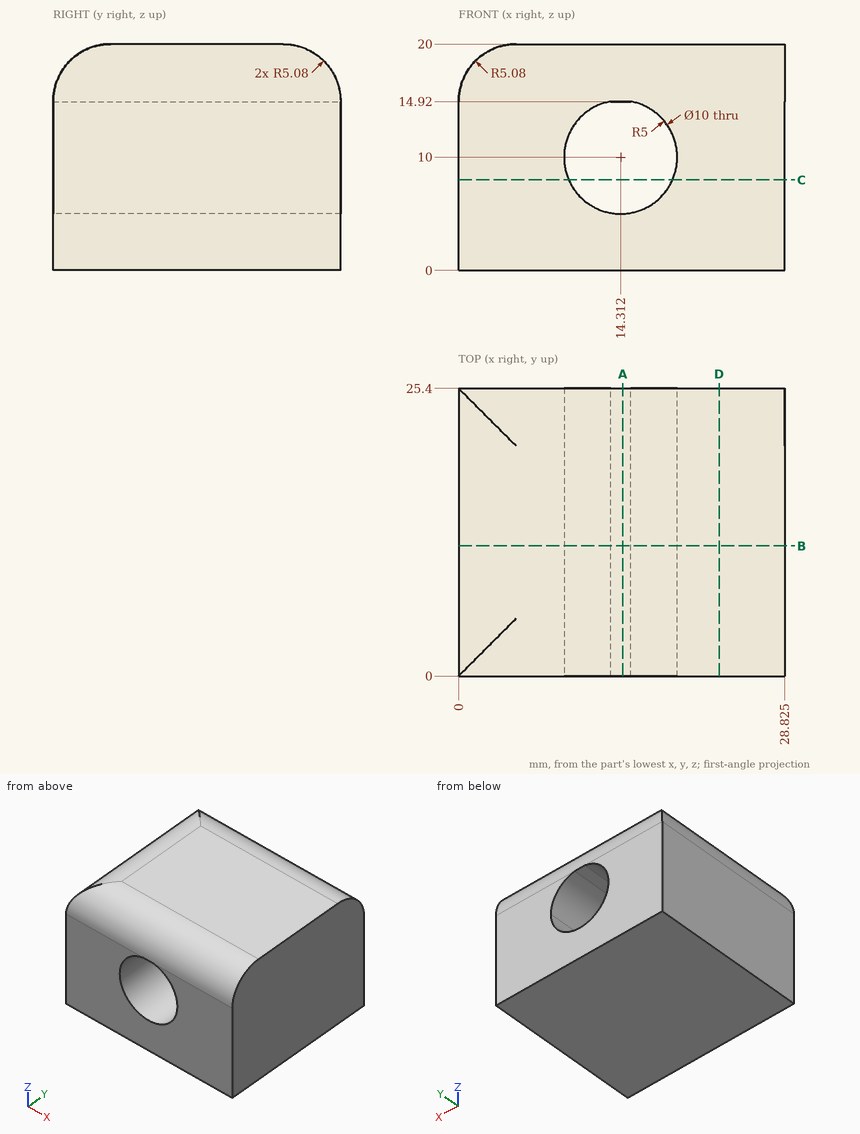
Answer from the drawing. Dimensions are ordinates in mm from the lowest x, y and z of the part. Give positions to 0.01 mm unless a question says otherwise; leave off trailing zeros. Loops run counter-clockwise (first coordinate to the right, second up) from the corner with the lowest first, then second, coordinate; pieces in that order, holes last. Notation, with made-up numbers: (21, 48.5) -> (59, 48.5) arc R21 ccw to (59, 58.5) -> close; hole circle Ø6 at (80.25, -3). An arc over 180 degrees is marked (long way). One line per question, with ' | ' between items. Start each with the question number.
1) Section B-B, the plane y = 11.5 is taken. Determine the outline of the cut face in (x, z) (1 decimal).
2) Section C-C, the plane z = 8 is taken. Determine the outline of the cut face in (x, y) (1 decimal), then the cut area to 3 significant figures.
3) Straight lines are drawn through the part: L1, parallel to X at y = 15.5, z = 10 (1 decimal); L2, parallel to Z at x = 14.25, y = 19.75; L3, parallel to X at y = 6, z = 6.75 (1 decimal). For each, find the intervals that lie inside material, in ascending order.
4) Section A-A, the plane x = 14.5 is taken. Determine the outline of the cut face in (y, z), then the cut area to 3 significant figures.
5) This flat-tipped pin is pushed along its axis until it touches: pin 1 (1.5 mm diameter, centred on y = 15, z = 17, fed in from -X). Where does it stop, or does it pass through?
6) Section D-D, the plane x = 23 is taken. Determine the outline of the cut face in (y, z).
Resolved:
1) outline: (0, 0) -> (28.8, 0) -> (28.8, 20) -> (5.1, 20) arc R5.1 ccw to (0, 14.9) -> close; hole (13.4, 14.9) arc R5 ccw (long way) to (15.2, 14.9) -> close
2) outline: (0, 0) -> (9.7, 0) -> (9.7, 25.4) -> (0, 25.4) -> close; (18.9, 0) -> (28.8, 0) -> (28.8, 25.4) -> (18.9, 25.4) -> close | area: 499 mm2
3) L1: 0 to 9.3, 19.3 to 28.8 | L2: 0 to 5, 14.92 to 20 | L3: 0 to 10.5, 18.1 to 28.8
4) outline: (0, 0) -> (25.4, 0) -> (25.4, 5) -> (0, 5) -> close; (0, 14.92) -> (25.4, 14.92) arc R5.08 ccw to (20.32, 20) -> (5.08, 20) arc R5.08 ccw to start | area: 245 mm2
5) pin 1: x = 0.18
6) outline: (0, 0) -> (25.4, 0) -> (25.4, 14.92) arc R5.08 ccw to (20.32, 20) -> (5.08, 20) arc R5.08 ccw to (0, 14.92) -> close
